Here's how the part is built. I have some questions about the finished solid (model axes, mm). Coordinates: 2 decimals unless noted, no trailing zeros. Write each loop counter-clockwise with the first axis right and the second up, starting at its lowest first coordinate (ties: lowest second). Pieces come first, ordered by that corner, then holes.
Item 1: I want a section at B-B (y = 1.15). Please give me the cut outline in (x, z), and give its area (3 significant figures).
Item 2: I want a section at A-A (z = 0). Please give me the cut outline in (x, y).
Item 3: Please list where these lines run through material, in increasing order: line 1 (X direction, y = 0.65, z = 1.5); line 2 (X direction, y = 0.1, z = -0.5).
Autodesk Inventor part; units mm, degrees
ref_plane "YZ Plane" through (0, 0, 0) normal (1, 0, 0) x (0, 1, 0)
ref_plane "XZ Plane" through (0, 0, 0) normal (0, 1, 0) x (-1, 0, 0)
ref_plane "XY Plane" through (0, 0, 0) normal (0, 0, 1) x (1, 0, 0)
sketch "Sketch1" plane through (0, 0, 0) normal (0, 1, 0) x (-1, 0, 0)
  line L0 (27.7495, 9.9695) -> (-27.7495, 9.9695)
  line L1 (-27.7495, 9.9695) -> (-27.7495, -9.9695)
  line L2 (-27.7495, -9.9695) -> (27.7495, -9.9695)
  line L3 (27.7495, -9.9695) -> (27.7495, 9.9695)
  line L4 (27.7495, 9.9695) -> (-27.7495, -9.9695) construction
  line L5 (-27.7495, 9.9695) -> (27.7495, -9.9695) construction
  circle A0 centre (25.7175, 0) radius 1.75
  circle A1 centre (-25.7175, 0) radius 1.75
  point P0 (0, 0)
  dimension "d0" = 55.499
  dimension "d1" = 19.939
  dimension "d2" = 3.5
  dimension "d3" = 3.5
  dimension "d4" = 2.032
  dimension "d5" = 2.032
extrude "Extrusion1" add sketch "Sketch1" along normal blind 1.7
sketch "Sketch2" plane through (0, 1.7, 0) normal (0, 1, 0) x (1, 0, 0)
  circle A0 centre (25.7175, 0) radius 1.75
  circle A1 centre (-25.7175, 0) radius 1.75
  line L0 (-27.7495, -9.9695) -> (27.7495, -9.9695)
  line L1 (27.7495, -9.9695) -> (27.7495, 9.9695)
  line L2 (27.7495, 9.9695) -> (-27.7495, 9.9695)
  line L3 (-27.7495, 9.9695) -> (-27.7495, -9.9695)
  line L4 (16.1881, -1.9444) -> (-16.645, -1.9444) construction
  line L5 (-16.645, -1.9444) -> (-16.645, 1.7031) construction
  line L6 (-16.645, 1.7031) -> (16.1881, 1.7031) construction
  line L7 (16.1881, 1.7031) -> (16.1881, -1.9444) construction
  point P0 (0, 0)
properties part number "Start Stop"
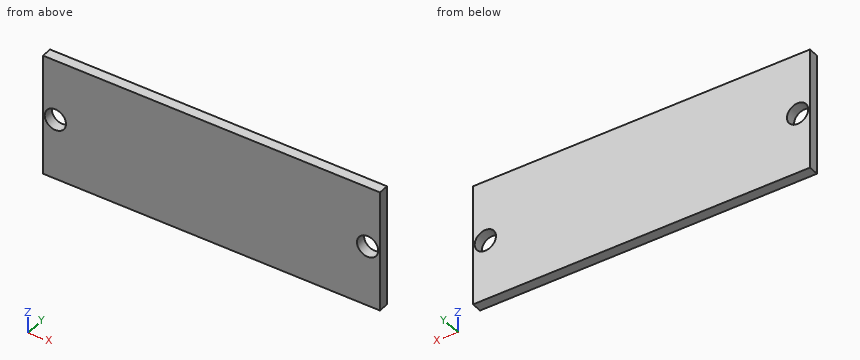
Answer:
1. outline: (-27.75, -9.97) - (27.75, -9.97) - (27.75, 9.97) - (-27.75, 9.97) - close; hole circle Ø3.5 at (-25.72, 0); hole circle Ø3.5 at (25.72, 0)
1. area: 1,090 mm2
2. outline: (-27.75, 0) - (-27.47, 0) - (-27.47, 1.7) - (-27.75, 1.7) - close; (-23.97, 0) - (23.97, 0) - (23.97, 1.7) - (-23.97, 1.7) - close; (27.47, 0) - (27.75, 0) - (27.75, 1.7) - (27.47, 1.7) - close
3. line 1: x = -27.75 to -26.62, -24.82 to 24.82, 26.62 to 27.75
3. line 2: x = -27.75 to -27.39, -24.04 to 24.04, 27.39 to 27.75
